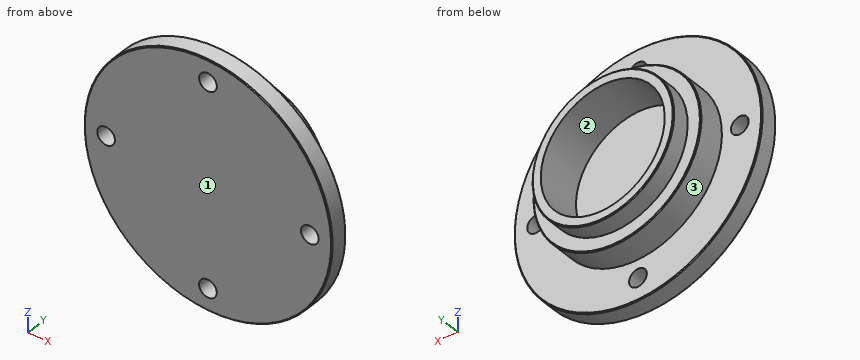
from build123d import *

# Parameters (mm, degrees)
SKETCH_1_R          = 47.4
EXTRUDE_1_DEPTH     = 15
SKETCH_2_R          = 40
EXTRUDE_2_DEPTH     = 10
SKETCH_3_R          = 70
SKETCH_3_R_2        = 5
EXTRUDE_3_DEPTH     = 10
SKETCH_4_R          = 35
CUT_EXTRUDE_1_DEPTH = 25
CHAMFER_1_SIZE      = 0.5


with BuildPart() as part:
    # 草图1 → 凸台-拉伸1 (new body)
    with BuildSketch(Plane(origin=(0, 0, 0), x_dir=(1, 0, 0), z_dir=(0, 1, 0))):
        with Locations(Location((0, 0, 0), (0, 0, 270))):
            Circle(SKETCH_1_R)
    extrude(amount=EXTRUDE_1_DEPTH)

    # 草图2 → 凸台-拉伸2 (add)
    with BuildSketch(Plane(origin=(0, 15, 0), x_dir=(1, 0, 0), z_dir=(0, 1, 0))):
        with Locations(Location((0, 0, 0), (0, 0, 270))):
            Circle(SKETCH_2_R)
    extrude(amount=EXTRUDE_2_DEPTH)

    # 草图3 → 凸台-拉伸3 (add)
    with BuildSketch(Plane.XZ):
        with Locations(Location((0, 0, 0), (0, 0, 270))):
            Circle(SKETCH_3_R)
        with Locations(Location((0, 57.5, 0), (0, 0, 270))):
            Circle(SKETCH_3_R_2, mode=Mode.SUBTRACT)
        with Locations(Location((57.5, 0, 0), (0, 0, 270))):
            Circle(SKETCH_3_R_2, mode=Mode.SUBTRACT)
        with Locations(Location((0, -57.5, 0), (0, 0, 270))):
            Circle(SKETCH_3_R_2, mode=Mode.SUBTRACT)
        with Locations(Location((-57.5, 0, 0), (0, 0, 270))):
            Circle(SKETCH_3_R_2, mode=Mode.SUBTRACT)
    extrude(amount=EXTRUDE_3_DEPTH)

    # 草图4 → 切除-拉伸1 (cut)
    with BuildSketch(Plane(origin=(0, 25, 0), x_dir=(1, 0, 0), z_dir=(0, 1, 0))):
        with Locations(Location((0, 0, 0), (0, 0, 270))):
            Circle(SKETCH_4_R)
    extrude(amount=-CUT_EXTRUDE_1_DEPTH, mode=Mode.SUBTRACT)

    # 倒角1
    chamfer_1_edges = [part.edges().sort_by_distance(p)[0] for p in [
        (0, 0, 70),
        (0, 15, -47.4),
        (0, 25, -40),
        (0, -10, 70),
    ]]
    chamfer(chamfer_1_edges, length=CHAMFER_1_SIZE)


solid = part.part
Model file for the job. Use its own axes, mm. Face numbers are marked on the shaded views. Give positions to 0.01 mm unless a question says otherwise; leave off trailing zeros. Write each loop counter-clockwise with the first axis right and the second up, starting at its lowest first coordinate (ties: lowest second). Pieces come first, ordered by that corner, then holes. Notation, with made-up numbers: M 30,24.25 L 61,24.25 A22 ccw 61,63.25 Z; hole C 37.5,-27.75 d11. An arc over 180 degrees is marked long. One line per item, written item: value. Start each with the question number.
Q1. Saw through at A-A, the plane z = 0. State how many separate pieces and enclosed holes the cut face has, plus the area to 3 significant figures.
Q2. Saw through at C-C, the plane y = 5. Write the cut outline in (x, z), plus the area to 3 significant figures.
Q3. Two-plate mould, pull along Z, no slides. Class the marked faces 1, 2 and 3: +Z half, -Z half, draft (parallel to the pull), parting line (faces both ways), or undercut.
Q4. Probe probe 1 along X at (y, z) = (-7, 0); probe 2 along X at (y, z) = (15.5, 0); probe 3 along X at (y, z) = (7, 20). List the from-to ranges inside material, lowest first. Write a range as [from, to].
Q5. Saw through at B-B, the plane y = 19.5. Write the cut outline in (x, z).
Q6. Drop flat-ended pins along their axis: pin 1 Ø16 at (x, z) = (57.5, 0) entering from +Y; pin 2 Ø1 at (y, z) = (-5, 14) entering from +X; pin 3 Ø2 at (x, y) = (-11.5, 13.5) entering from -Z. Give the stop position or say it passes through.
Output values:
1. separate pieces: 3
1. enclosed holes: 0
1. area: 1,670 mm²
2. outline: C 0,0 d94.8; hole C 0,0 d70
2. area: 3,210 mm²
3. face 1: draft
3. face 2: undercut
3. face 3: parting line
4. probe 1: x = [-70, -62.5], [-52.5, 52.5], [62.5, 70]
4. probe 2: x = [-40, -35], [35, 40]
4. probe 3: x = [-42.97, -28.72], [28.72, 42.97]
5. outline: C 0,0 d80; hole C 0,0 d70
6. pin 1: stops at y = 0
6. pin 2: stops at x = 68.69
6. pin 3: stops at z = -46.22
